from build123d import *

# Parameters (mm, degrees)
RADYUS1_R = 1.016


with BuildPart() as part:
    # Sketch1 → Döndür1 (revolve)
    with BuildSketch(Plane.XY, mode=Mode.PRIVATE) as d_nd_r1_sk:
        Polygon((6.35, -12.7), (9.525, -12.7), (9.525, 0), (14.2875, 0), (14.2875, 12.7), (11.1125, 12.7), (11.1125, 6.35), (6.35, 1.5875), align=None)
    revolve(d_nd_r1_sk.sketch.rotate(Axis((0, 0, 0), (0, 1, 0)), 90), axis=Axis((0, 0, 0), (0, 1, 0)))

    # Radyus1
    radyus1_edges = [part.edges().sort_by_distance(p)[0] for p in [
        (0, 1.5875, 6.35),
        (0, 12.7, 11.1125),
        (0, 12.7, 14.2875),
        (0, 0, 14.2875),
        (0, -12.7, 9.525),
    ]]
    fillet(radyus1_edges, radius=RADYUS1_R)


solid = part.part
The model under review builds one solid part; all positions refer to its coordinate system, in mm. A direction names the side the tool comes from. Round coordinates to 2 decimals unless told otherwise and drop trailing zeros. Write each loop counter-clockwise with the first axis right and the second up, starting at its lowest first coordinate (ties: lowest second). Pieces come first, ordered by that corner, then holes. Notation, with made-up numbers: M -4.75,-5.75 L 51.25,-5.75 A20 cw 51.25,9.25 Z; hole C -28.75,-39.75 d10. An arc over 180 degrees is marked long. Use a Markdown table: item, result. Add a question column.
Q1. To check wall thickness, follow line 1 (X direction, y = -6.75, z = 0) (3 decimals); line 2 (Y direction, x = 11.25, z = -5); line 3 (X direction, y = 9.2, z = 0). State the ranges of each line that lie inside material, in increasing order.
Q2. The part is to be moulded in two halves that separate along Z. For faces 1 (the face through (9.3, -5.76, 2.06)), 2 (the face through (3.86, -5.86, 5.04)), 3 (the face through (11, 12.7, -6)), say which applies: pulls with the +Z half, pulls with the -Z half, needs draft (parallel to the pull), parting line crosses it, or undercut.
Q3. Insertion check: pin 1 (4 mm diameter, centred on y = -10, z = -9.5, fed in from -X); pin 2 (1 mm diameter, centred on x = 2.5, y = 8.5, fed in from -Z); pin 3 (12 mm diameter, centred on y = 2, z = 6.5, fed in from +X). Each pin has a flat end and moves straight along its axis. Give the tip position at first contact, or say it passes through.
Q4. We need section A-A, the plane y = 9.75. State the section outline as (x, z) points (1 decimal).
Q5. Machinability: for faces 4 (the face through (6, -12.7, -3)), 5 (the face through (6, 0, 9)), 6 (the face through (-7.5, 9, 8.2)), which of the approach directions +Z, -Z, +X, -X, +Y, -Y give a long, thin tool a straight path to every point of the face, cutting with its end or side? Answer none if there is none.
Findings below:
| question | item | result |
|---|---|---|
| 1 | line 1 | x = -9.525 to -6.35, 6.35 to 9.525 |
| 1 | line 2 | y = 0 to 12.7 |
| 1 | line 3 | x = -14.29 to -11.11, 11.11 to 14.29 |
| 2 | face 1 | parting line crosses it |
| 2 | face 2 | undercut |
| 2 | face 3 | needs draft |
| 3 | pin 1 | stops at x = -5.87 |
| 3 | pin 2 | stops at z = -14.15 |
| 3 | pin 3 | stops at x = 14.28 |
| 4 | outline | C 0,0 d28.6; hole C 0,0 d22.2 |
| 5 | face 4 | +Z, -Z, +X, -X, -Y |
| 5 | face 5 | -Y |
| 5 | face 6 | +Y |
